```python
from build123d import *

# Parameters (mm, degrees)
SKETCH1_R           = 1
BOSS_EXTRUDE1_DEPTH = 50
SKETCH2_W           = 10
SKETCH2_H           = 2
BOSS_EXTRUDE2_DEPTH = 2
BOSS_EXTRUDE3_DEPTH = 2
CUT_EXTRUDE1_REACH  = 55.16
SKETCH5_R           = 0.45
BOSS_EXTRUDE4_DEPTH = 5


with BuildPart() as part:
    # Sketch1 → Boss-Extrude1 (new body)
    with BuildSketch(Plane.XY):
        Circle(SKETCH1_R)
    extrude(amount=BOSS_EXTRUDE1_DEPTH)

    # Sketch2 → Boss-Extrude2 (add)
    with BuildSketch(Plane.XY.offset(50)):
        with Locations((5, 0)):
            Rectangle(SKETCH2_W, SKETCH2_H)
    extrude(amount=BOSS_EXTRUDE2_DEPTH)

    # Sketch3 → Boss-Extrude3 (add)
    with BuildSketch(Plane.XY.offset(50)):
        with BuildLine():
            Line((0, -1), (0, 1))
            ThreePointArc((0, 1), (-1, 0), (0, -1))
        make_face()
    extrude(amount=BOSS_EXTRUDE3_DEPTH)

    # Sketch4 → Cut-Extrude1 (cut, up to next)
    with BuildSketch(Plane(origin=(10, 0, 0), x_dir=(0, 0, -1), z_dir=(1, 0, 0)), mode=Mode.PRIVATE) as cut_extrude1_sk1:
        with BuildLine():
            ThreePointArc((-52, 0), (-51.707106781, 0.707106781), (-51, 1))
            Line((-51, 1), (-52, 1))
            Line((-52, 1), (-52, 0))
        make_face()
    cut_extrude1_tool1 = extrude(cut_extrude1_sk1.sketch, amount=-CUT_EXTRUDE1_REACH, mode=Mode.PRIVATE) & part.part
    # Sketch4 → Cut-Extrude1 (cut, up to next)
    with BuildSketch(Plane(origin=(10, 0, 0), x_dir=(0, 0, -1), z_dir=(1, 0, 0)), mode=Mode.PRIVATE) as cut_extrude1_sk2:
        with BuildLine():
            Line((-52, -1), (-51, -1))
            ThreePointArc((-51, -1), (-51.707106781, -0.707106781), (-52, 0))
            Line((-52, 0), (-52, -1))
        make_face()
    cut_extrude1_tool2 = extrude(cut_extrude1_sk2.sketch, amount=-CUT_EXTRUDE1_REACH, mode=Mode.PRIVATE) & part.part
    add(cut_extrude1_tool1.solids().sort_by_distance((10, 0.776632, 51.776632))[0], mode=Mode.SUBTRACT)
    add(cut_extrude1_tool2.solids().sort_by_distance((10, -0.776632, 51.776632))[0], mode=Mode.SUBTRACT)

    # Sketch5 → Boss-Extrude4 (add)
    with BuildSketch(Plane(origin=(0, 0, 0), x_dir=(-1, 0, 0), z_dir=(0, 0, -1))):
        with Locations(Location((0.5, 0, 0), (0, 0, 180))):
            Circle(SKETCH5_R)
        with Locations(Location((-0.5, 0, 0), (0, 0, 180))):
            Circle(SKETCH5_R)
    extrude(amount=BOSS_EXTRUDE4_DEPTH)


solid = part.part
```
Geometry: final body of the model. Coordinates: model frame, mm. A direction names the side the tool comes from. Round coordinates to 2 decimals unless told otherwise and drop trailing zeros. Loops run counter-clockwise (first coordinate to the right, second up) from the corner with the lowest first, then second, coordinate; pieces in that order, holes last. Notation, with made-up numbers: (55, 45) -> (96, 45) arc R22 cw to (96, 74) -> close; hole circle Ø8 at (10.25, 35.25). An arc over 180 degrees is marked (long way). Use one line per item in the form item = value. Start each with the question number.
1) Access query for faces 5 (the flat face through (0.5, 0, -5)), 6 (the cylindrical face through (0.929, -0.135, -2.465)). Directions: +Z, -Z, +X, -X, +Y, -Y. A direction counts if a zero-diameter tool reaches every point of the face in a straight line with its end or side. Return the directions, or none.
2) Section A-A on x = 6. Output: boundary loops of the cut face in (y, z).
3) Section B-B on z = 19.5. Output: boundary loops of the cut face in (x, y).
4) Line query: L1, parallel to X at y = -0.85, z = 29; L2, parallel to X at y = 0.35, z = 3.5; L3, parallel to Z at x = 9.5, y = -0.05. Output: solid intervals per line, ascending.
5) Draft query along X for faces 1 (the flat face through (4.9, 1, 50.5)), 2 (the cylindrical face through (-0.29, 0.4, -2.46)), 3 (the flat face through (10, 0, 51)), 4 (the cylindrical face through (0, -1, 26)). Return one class per face: released by +X, released by -X, zero draft, split by the parting line, or undercut.
Response:
q1.face_5 = -Z, +X, -X, +Y, -Y
q1.face_6 = -Z
q2.outline = (-1, 50) -> (1, 50) -> (1, 51) arc R1 ccw to (-1, 51) -> close
q3.outline = circle Ø2 at (0, 0)
q4.L1 = -0.53 to 0.53
q4.L2 = -0.94 to 0.94
q4.L3 = 50 to 52
q5.face_1 = zero draft
q5.face_2 = undercut
q5.face_3 = released by +X
q5.face_4 = split by the parting line
